```python
from build123d import *

# Parameters (mm, degrees)
CUT_EXTRUDE1_DEPTH      = 18
CUT_EXTRUDE1_DEPTH_BACK = 18
SKETCH2_R               = 2.1
SKETCH3_W               = 9
SKETCH3_H               = 9
CUT_EXTRUDE4_DEPTH      = 3.1
SKETCH4_W               = 9
SKETCH4_H               = 9
SKETCH4_R               = 2.1
BOSS_EXTRUDE2_DEPTH     = 1
BOSS_EXTRUDE3_START     = -1.850787983
BOSS_EXTRUDE3_DEPTH     = 0.850787983
FILLET2_R               = 3
CUT_EXTRUDE5_DEPTH      = 3
SKETCH9_W               = 10
SKETCH9_H               = 7.5
SKETCH9_R               = 2.1
CUT_EXTRUDE6_DEPTH      = 2.75
SKETCH10_R              = 2.1
CUT_EXTRUDE7_DEPTH      = 37.75
SKETCH11_R              = 3.5
CUT_EXTRUDE8_DEPTH      = 17
SKETCH12_R              = 3.5
CUT_EXTRUDE9_DEPTH      = 4


# Read off the part's stored shape, not the designer's step: Boss-Extrude3
with BuildPart() as part:
    # Sketch1 → Revolve2 (revolve)
    with BuildSketch(Plane.XY, mode=Mode.PRIVATE) as revolve2_sk:
        with BuildLine():
            Line((0, 27.5), (0, 16))
            ThreePointArc((0, 16), (4.539948066, 14.894753), (7.995845625, 11.75))
            Line((7.995845625, 11.75), (9.755894266, 7.4))
            Line((9.755894266, 7.4), (12.75, 0))
            Line((12.75, 0), (14.75, 0))
            Line((14.75, 0), (7.7, 27.5))
            Line((7.7, 27.5), (0, 27.5))
        make_face()
    revolve(revolve2_sk.sketch.rotate(Axis((0, 27.5, 0), (0, -1, 0)), 90), axis=Axis((0, 27.5, 0), (0, -1, 0)))

    # Sketch2 → Cut-Extrude1 (cut, two sides: drawn at the far end of the back side and taken through both)
    with BuildSketch(Plane(origin=(0, 0, 0), x_dir=(0, 0, -1), z_dir=(1, 0, 0)).offset(-CUT_EXTRUDE1_DEPTH_BACK)):
        with Locations(Location((0, 7.4, 0), (0, 0, 322.555636433))):
            Circle(SKETCH2_R)
    extrude(amount=CUT_EXTRUDE1_DEPTH + CUT_EXTRUDE1_DEPTH_BACK, mode=Mode.SUBTRACT)

    # Sketch3 → Cut-Extrude4 (cut)
    with BuildSketch(Plane(origin=(14.75, 0, 0), x_dir=(0, 0, -1), z_dir=(1, 0, 0))):
        with Locations((0, 7.4)):
            Rectangle(SKETCH3_W, SKETCH3_H)
    extrude(amount=-CUT_EXTRUDE4_DEPTH, mode=Mode.SUBTRACT)

    # Sketch4 → Boss-Extrude2 (add)
    with BuildSketch(Plane(origin=(11.65, 0, 0), x_dir=(0, 0, -1), z_dir=(1, 0, 0))):
        with Locations((0, 7.4)):
            Rectangle(SKETCH4_W, SKETCH4_H)
        with Locations(Location((0, 7.4, 0), (0, 0, 328.733960859))):
            Circle(SKETCH4_R, mode=Mode.SUBTRACT)
    extrude(amount=BOSS_EXTRUDE2_DEPTH)

    # Boss-Extrude3 outline → Boss-Extrude3 (add)
    with BuildSketch(Plane(origin=(12.65, 0, 0), x_dir=(0, 0, -1), z_dir=(1, 0, 0)).offset(BOSS_EXTRUDE3_START)):
        with BuildLine():
            Line((1.769303732, 8.531178281), (4.5, 8.531178281))
            Line((4.5, 8.531178281), (4.5, 11.9))
            Line((4.5, 11.9), (-4.5, 11.9))
            Line((-4.5, 11.9), (-4.5, 8.531178281))
            Line((-4.5, 8.531178281), (-1.769303732, 8.531178281))
            ThreePointArc((-1.769303732, 8.531178281), (0, 9.5), (1.769303732, 8.531178281))
        make_face()
    extrude(amount=BOSS_EXTRUDE3_DEPTH)

    # Fillet2
    fillet2_edges = [part.edges().sort_by_distance(p)[0] for p in [
        (11.724606008, 11.9, -4.5),
        (11.724606008, 11.9, 4.5),
    ]]
    fillet(fillet2_edges, radius=FILLET2_R)

    # Sketch8 → Cut-Extrude5 (cut)
    with BuildSketch(Plane(origin=(-14.75, 0, 0), x_dir=(0, 0, -1), z_dir=(1, 0, 0))):
        Polygon((3.6, 5.3), (3.6, 9.5), (0, 11.5), (-3.6, 9.5), (-3.6, 5.3), (0, 3.3), align=None)
    extrude(amount=CUT_EXTRUDE5_DEPTH, mode=Mode.SUBTRACT)

    # Sketch9 → Cut-Extrude6 (cut)
    # profile 1 of 3: a face of its own
    with BuildSketch(Plane(origin=(0, 27.5, 0), x_dir=(1, 0, 0), z_dir=(0, 1, 0))):
        with BuildLine():
            Line((-5, -3.75), (-5, 3.75))
            ThreePointArc((-5, 3.75), (-5.933352987, 0), (-5, -3.75))
        make_face()
    # profile 2 of 3: a face of its own
    with BuildSketch(Plane(origin=(0, 27.5, 0), x_dir=(1, 0, 0), z_dir=(0, 1, 0))):
        Rectangle(SKETCH9_W, SKETCH9_H)
        with Locations(Location((0, 0, 0), (0, 0, 270))):
            Circle(SKETCH9_R, mode=Mode.SUBTRACT)
    # profile 3 of 3: a face of its own
    with BuildSketch(Plane(origin=(0, 27.5, 0), x_dir=(1, 0, 0), z_dir=(0, 1, 0))):
        with BuildLine():
            ThreePointArc((5, 3.75), (5.933352987, 0), (5, -3.75))
            Line((5, -3.75), (5, 3.75))
        make_face()
    extrude(amount=-CUT_EXTRUDE6_DEPTH, mode=Mode.SUBTRACT)

    # Sketch10 → Cut-Extrude7 (cut)
    with BuildSketch(Plane(origin=(0, 27.5, 0), x_dir=(1, 0, 0), z_dir=(0, 1, 0))):
        with Locations(Location((0, 0, 0), (0, 0, 270))):
            Circle(SKETCH10_R)
    extrude(amount=-CUT_EXTRUDE7_DEPTH, mode=Mode.SUBTRACT)

    # Sketch11 → Cut-Extrude8 (cut)
    with BuildSketch(Plane(origin=(0, 0, 0), x_dir=(-1, 0, 0), z_dir=(0, -1, 0))):
        with Locations(Location((0, 0, 0), (0, 0, 90))):
            Circle(SKETCH11_R)
    extrude(amount=-CUT_EXTRUDE8_DEPTH, mode=Mode.SUBTRACT)

    # Sketch12 → Cut-Extrude9 (cut)
    with BuildSketch(Plane(origin=(0, 17, 0), x_dir=(-1, 0, 0), z_dir=(0, -1, 0))):
        with Locations(Location((0, 0, 0), (0, 0, 90))):
            Circle(SKETCH12_R)
    extrude(amount=-CUT_EXTRUDE9_DEPTH, mode=Mode.SUBTRACT)


solid = part.part
```
Input: part model. Units: mm. Frame: model coordinates. A direction names the side the tool comes from. Round coordinates to 2 decimals unless told otherwise and drop trailing zeros. Loops run counter-clockwise (first coordinate to the right, second up) from the corner with the lowest first, then second, coordinate; pieces in that order, holes last.
1) Set-up query: faces 4 (the cylindrical face through (12.01, 11, 3.64)), 5 (the flat face through (0, 26, 3.75)), 6 (the cylindrical face through (12.01, 11.04, -3.6)). Return all of +Z, -Z, +X, -X, +Y, -Y with unobstructed straight access to the full face (end or side cutting, diameter ignored); none if empty.
Ans:
face 4: +Z, +X, +Y
face 5: +Y
face 6: -Z, +X, +Y
2) Pin query (flat end, axial travel): pin 1 (6.5 mm diameter, centred on y = 7.4, z = 0, fed in from -X); pin 2 (0.5 mm diameter, centred on x = 13, y = 3.5, fed in from +Z); pin 3 (0.5 mm diameter, centred on x = 12, y = 6.5, fed in from +Z). Return the tip coordinate at first contact, or that it passes through.
Ans:
pin 1: stops at x = -11.75
pin 2: stops at z = 5.44
pin 3: stops at z = 5.78
3) Section query B-B on y = 17. Return the cut outline in (x, z).
Ans:
outline: circle Ø20.78 at (0, 0); hole circle Ø7 at (0, 0)
4) Section query A-A on y = 4.75. Return the cut outline in (x, z).
Ans:
outline: (-13.28, -2.61) arc R13.53 ccw to (12.76, -4.5) - (12.65, -4.5) - (12.65, 4.5) - (12.76, 4.5) arc R13.53 ccw to (-13.28, 2.61) - (-11.75, 2.61) - (-11.75, -2.61) - close; hole circle Ø21.66 at (0, 0)
5) Pull-direction query (X, two-part tool) for faces 1 (the conical face through (-8.76, 17, 5.59)), 2 (the flat face through (-12.6, 4.3, -1.8)), 3 (the cylindrical face through (0.631, 22.901, 2.003)); classes: released by +X, released by -X, zero draft, split by the parting line, or undercut.
Ans:
face 1: split by the parting line
face 2: zero draft
face 3: undercut
6) Material intervals for line 1 (Y direction, x = -2.5, z = 1); line 2 (X direction, y = 18.75, z = -1.5); line 3 (X direction, y = 3.75, z = 6), sorted ascending.
Ans:
line 1: y = 21 to 24.75
line 2: x = -9.83 to -3.16, 3.16 to 9.83
line 3: x = -12.41 to -9.5, 9.5 to 12.41
